from build123d import *

# Parameters (mm, degrees)
F0_W     = 101.6
F0_H     = 101.6
F1_DEPTH = 50.8
F2_R     = 25.4
F3_DEPTH = 38.1
F4_R     = 12.7
F5_SIZE  = 2.54
F6_SIZE  = 6.35


with BuildPart() as f1:
    # F0 (on Top) → F1 (new body)
    with BuildSketch(Plane.XY):
        with Locations((50.8, 50.8)):
            Rectangle(F0_W, F0_H)
    extrude(amount=F1_DEPTH)

    # F2 (on face) → F3 (cut)
    with BuildSketch(Plane.XY.offset(50.8)):
        with Locations((50.8, 50.8)):
            Circle(F2_R)
    extrude(amount=-F3_DEPTH, mode=Mode.SUBTRACT)

    # F4
    f4_edges = [f1.edges().sort_by_distance(p)[0] for p in [
        (101.6, 0, 25.4),
        (0, 0, 25.4),
        (101.6, 101.6, 25.4),
        (0, 101.6, 25.4),
    ]]
    fillet(f4_edges, radius=F4_R)

    # F5
    f5_edges = [f1.edges().sort_by_distance(p)[0] for p in [
        (25.4, 50.8, 12.7),
        (25.4, 50.8, 50.8),
    ]]
    chamfer(f5_edges, length=F5_SIZE)

    # F6
    f6_edges = [f1.edges().sort_by_distance(p)[0] for p in [
        (0, 50.8, 50.8),
    ]]
    chamfer(f6_edges, length=F6_SIZE)


solid = f1.part
Source: CAD feature listing. Evaluate the final solid. Frame: model axes, mm. A direction names the side the tool comes from. Give positions to 0.01 mm unless a question says otherwise; leave off trailing zeros. Order: outer loops, then holes, each group sorted by start corner. A loop starts at its lowest first (then second) coordinate and runs counter-clockwise, first axis right, second up. Notation, with made-up numbers: (43, 71) -> (76, 71) arc R10 cw to (76, 88) -> close; hole circle Ø5 at (-8, 81). An arc over 180 degrees is marked (long way). Write item = value, one per line.
Item 1: Mould query, pull axis Y, two halves, no side actions, for faces 1 (the face through (50, 101.6, 22)), 2 (the face through (30.5, 35.3, 48.4)), 3 (the face through (50, 0, 22)), 4 (the face through (30, 71, 50.8)). Classes: +Y half, -Y half, draft (parallel to the pull), parting line (faces both ways), or undercut.
Check result:
face_1 = +Y half
face_2 = undercut
face_3 = -Y half
face_4 = draft
Item 2: Set-up query: faces 5 (the face through (3.62, 3.82, 22.54)), 6 (the face through (50, 51, 12.7)). Return all of +Z, -Z, +X, -X, +Y, -Y with unobstructed straight access to the full face (end or side cutting, diameter ignored); none if empty.
Check result:
face_5 = +Z, -Z, -X, -Y
face_6 = +Z
Item 3: Section query B-B (y = 50.8). Output: boundary loops of the cut face in (x, z), then the cut area to 3 significant figures.
Check result:
outline = (0, 0) -> (101.6, 0) -> (101.6, 44.45) -> (95.25, 50.8) -> (78.74, 50.8) -> (76.2, 48.26) -> (76.2, 15.24) -> (73.66, 12.7) -> (27.94, 12.7) -> (25.4, 15.24) -> (25.4, 48.26) -> (22.86, 50.8) -> (6.35, 50.8) -> (0, 44.45) -> close
area = 3,190 mm²
Item 4: Ray query, probe 1 along Y at (x, z) = (50.8, 29.5); probe 2 along X at (y, z) = (50, 29); probe 3 along X at (y, z) = (33, 35.5). Return the intervals inside material, ascending.
Check result:
probe_1 = 0 to 25.4, 76.2 to 101.6
probe_2 = 0 to 25.41, 76.19 to 101.6
probe_3 = 0 to 32.68, 68.92 to 101.6
Item 5: Contact query for flat-ended pins moving along their axis: pin 1 (8 mm diameter, centred on x = 69.5, y = 36, fed in from +Z); pin 2 (23 mm diameter, centred on x = 43.5, y = 44.5, fed in from +Z). Output: stop coordinate, or through.
Check result:
pin_1 = 50.71
pin_2 = 12.7
Item 6: Section query A-A (z = 32). Output: boundary loops of the cut face in (x, y).
Check result:
outline = (0, 12.7) arc R12.7 ccw to (12.7, 0) -> (88.9, 0) arc R12.7 ccw to (101.6, 12.7) -> (101.6, 88.9) arc R12.7 ccw to (88.9, 101.6) -> (12.7, 101.6) arc R12.7 ccw to (0, 88.9) -> close; hole circle Ø50.8 at (50.8, 50.8)
